Part print with two shaded views. Sizes in mm from the minimum x, y, z corner. A direction names the side the tool comes from. Give positions to 0.01 mm unless a question says otherwise; leave off trailing zeros. Write each loop counter-clockwise with the first axis right and the second up, starting at its lowest first coordinate (ties: lowest second). Pieces come first, ordered by that corner, then holes. Notation, with made-up numbers: M 77,80 L 116,80 A28 cw 116,111 Z; hole C 59.25,81 d3. An arc over 180 degrees is marked long. Return JSON: item names as keys, results as strings. Group by question number.
Q1. Wall check: probe 1 along X at (y, z) = (5, 32.5); probe 2 along X at (y, z) = (20.5, 21); probe 3 along Z at (x, y) = (19, 4.5). Give the ranges that are in metal, low to high.
Q2. Band-saw the part on C-C, the plane x = 10.5. Give the cut face in (y, z).
Q3. Tool access for the marked faces 1, 2 and 3: list every direction of +Z, -Z, +X, -X, +Y, -Y with a clear straight run to the whole face (end or side of a thin tool).
Q4. Band-saw the part on B-B, the plane z = 12. Give the cut face in (x, y), then the cut area to 3 significant figures.
Q5. Band-saw the part on A-A, the plane y = 27. Give the cut face in (x, z).
Q6. Flat gauge pins, fed straight in: pin 1 Ø5 at (x, y) = (23, 8.5) entering from +Z; pin 2 Ø0.8 at (x, z) = (32.5, 23) entering from +Y; pin 3 Ø6 at (x, z) = (9.5, 21) entering from +Y; pin 4 Ø5.5 at (y, z) = (14.5, 20.5) entering from -X. Where does each tip first touch, or does it go through?
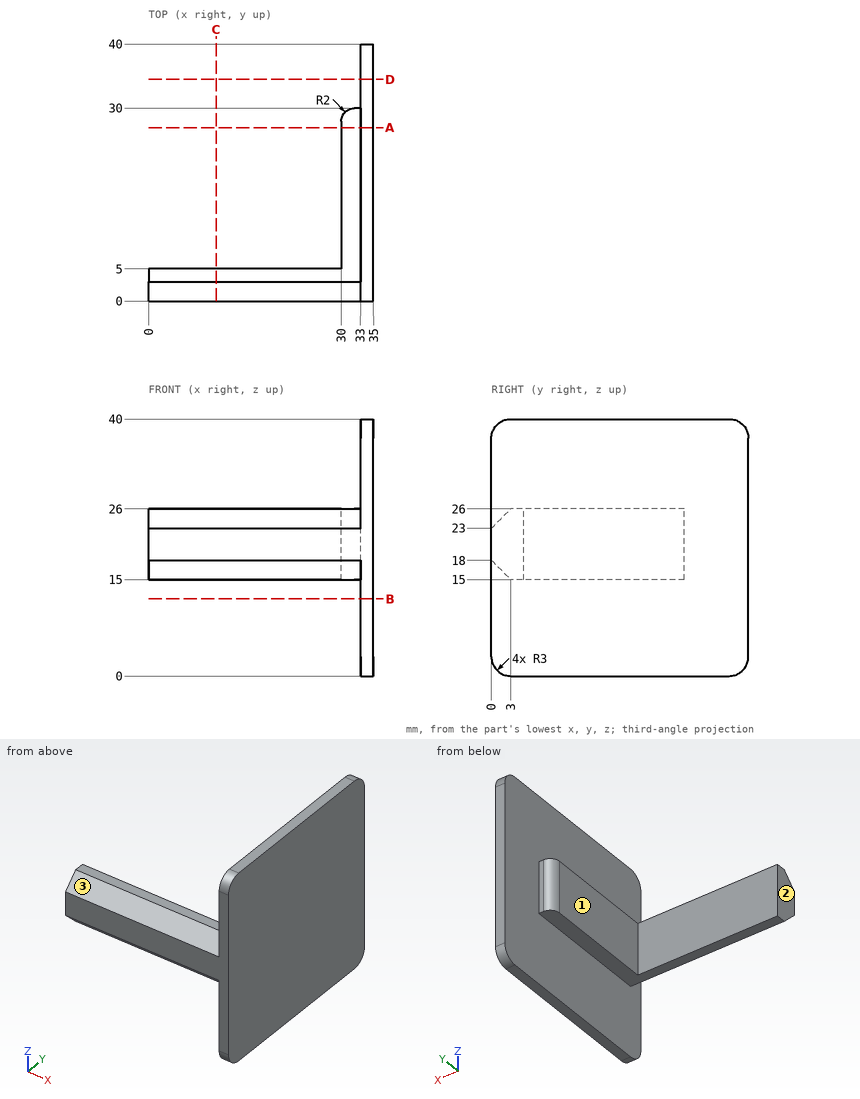
From the geometry:
{
 "1": {"probe 1": "x = 33 to 35", "probe 2": "x = 30 to 35", "probe 3": "z = 15 to 26"},
 "2": {"outline": "M 0,18 L 3,15 L 5,15 L 5,26 L 3,26 L 0,23 Z"},
 "3": {"face 1": "+Z, -Z, -X, +Y", "face 2": "+Z, -Z, -X, +Y, -Y", "face 3": "+Z, -X, -Y"},
 "4": {"outline": "M 33,0 L 35,0 L 35,40 L 33,40 Z", "area": "80.0 mm^2"},
 "5": {"outline": "M 30,15 L 33,15 L 33,0 L 35,0 L 35,40 L 33,40 L 33,26 L 30,26 Z"},
 "6": {"pin 1": "passes through", "pin 2": "stops at y = 30", "pin 3": "stops at y = 5", "pin 4": "stops at x = 30"}
}
